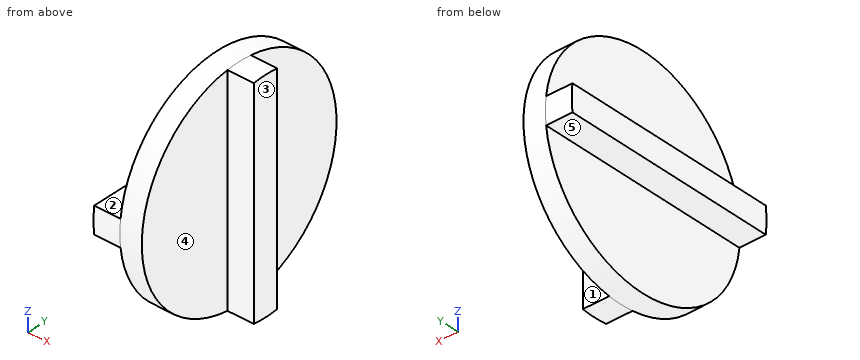
from build123d import *
from build123d.topology import SkipClean

# Parameters (mm, degrees)
SKETCH1_R           = 50
BOSS_EXTRUDE1_DEPTH = 10
BOSS_EXTRUDE2_DEPTH = 12
BOSS_EXTRUDE3_START = 12
BOSS_EXTRUDE3_DEPTH = 12


with BuildPart() as part:
    # Sketch1 → Boss-Extrude1 (new body)
    with BuildSketch(Plane(origin=(0, 0, 0), x_dir=(0, 0, -1), z_dir=(1, 0, 0))):
        Circle(SKETCH1_R)
    extrude(amount=BOSS_EXTRUDE1_DEPTH)

    # Sketch2 → Boss-Extrude2 (add)
    with SkipClean():  # the faces are left unmerged after this step: merging them gives an invalid solid
        with BuildSketch(Plane(origin=(10, 0, 0), x_dir=(0, 0, -1), z_dir=(1, 0, 0))):
            with BuildLine():
                Line((-49.638694584, 6), (49.638694584, 6))
                ThreePointArc((49.638694584, 6), (50, 0), (49.638694584, -6))
                Line((49.638694584, -6), (-49.638694584, -6))
                ThreePointArc((-49.638694584, -6), (-50, 0), (-49.638694584, 6))
            make_face()
        extrude(amount=BOSS_EXTRUDE2_DEPTH)

    # Sketch3 → Boss-Extrude3 (add)
    with SkipClean():  # the faces are left unmerged after this step: merging them gives an invalid solid
        with BuildSketch(Plane.ZY.offset(BOSS_EXTRUDE3_START)):
            with BuildLine():
                ThreePointArc((6, 49.638694584), (0, 50), (-6, 49.638694584))
                Line((-6, 49.638694584), (-6, -49.638694584))
                ThreePointArc((-6, -49.638694584), (0, -50), (6, -49.638694584))
                Line((6, -49.638694584), (6, 49.638694584))
            make_face()
        extrude(amount=-BOSS_EXTRUDE3_DEPTH)


solid = part.part
CAD build for the part. Positions are in the model's coordinates, mm. Face numbers are marked on the shaded views. A direction names the side the tool comes from. Give positions to 0.01 mm unless a question says otherwise; leave off trailing zeros. Loops run counter-clockwise (first coordinate to the right, second up) from the corner with the lowest first, then second, coordinate; pieces in that order, holes last. Notation, with made-up numbers: M 63.5,65 L 105.5,65 A17 cw 105.5,78 Z; hole C 22.5,61.25 d10. An arc over 180 degrees is marked long. One line per question, with ' | ' between items. Start each with the question number.
1. Saw through at C-C on x = 12. Give the cut face in (y, z).
2. Saw through at B-B on z = -36. Give the cut face in (x, y).
3. Saw through at A-A on y = 30. Give the cut face in (x, z), plus the area to 3 significant figures.
4. 3-axis set-ups, long thin cutter, end or side, ignore diameter. For the marked faces 1, 2, 3, 4 and 5: which of +Z, -Z, +X, -X, +Y, -Y reach the whole face in a straight line?
5. Flat gauge pins, fed straight in: pin 1 (10 mm diameter, centred on x = 0, y = -25, fed in from -Z); pin 2 (10 mm diameter, centred on x = -8, y = 6.5, fed in from -Z); pin 3 (6 mm diameter, centred on x = 13.5, z = -19.5, fed in from +Y). Where does each tip first touch, or does it go through?
6. Probe L1, parallel to X at y = 23, z = 21; L2, parallel to Z at x = 1, y = 0.5; L3, parallel to Y at x = 15, z = 28.5. List the from-to ranges inside material, lowest first. Write a range as from..to.
Result sheet:
1) outline: M -6,-49.64 A50 ccw 6,-49.64 L 6,49.64 A50 ccw -6,49.64 Z
2) outline: M 0,-34.7 L 10,-34.7 L 10,-6 L 22,-6 L 22,6 L 10,6 L 10,34.7 L 0,34.7 Z
3) outline: M -12,-6 L 0,-6 L 0,-40 L 10,-40 L 10,40 L 0,40 L 0,6 L -12,6 Z | area: 944 mm^2
4) face 1: +Z, -Z, +X, +Y | face 2: +Z, -X, +Y, -Y | face 3: +Z, -Z, +X, +Y, -Y | face 4: +Z, -Z, +X, -Y | face 5: -Z, -X, +Y, -Y
5) pin 1: stops at z = -45.83 | pin 2: stops at z = -6 | pin 3: stops at y = 6
6) L1: x = 0..10 | L2: z = -50..50 | L3: y = -6..6
